Answer from the drawing. Dimensions are ordinates in mm from the lowest x, y and z of the part. Round coordinates to 2 decimals unless told otherwise and drop trailing zeros. Loops run counter-clockwise (first coordinate to the right, second up) from the corner with the lowest first, then second, coordinate; pieces in that order, holes last.
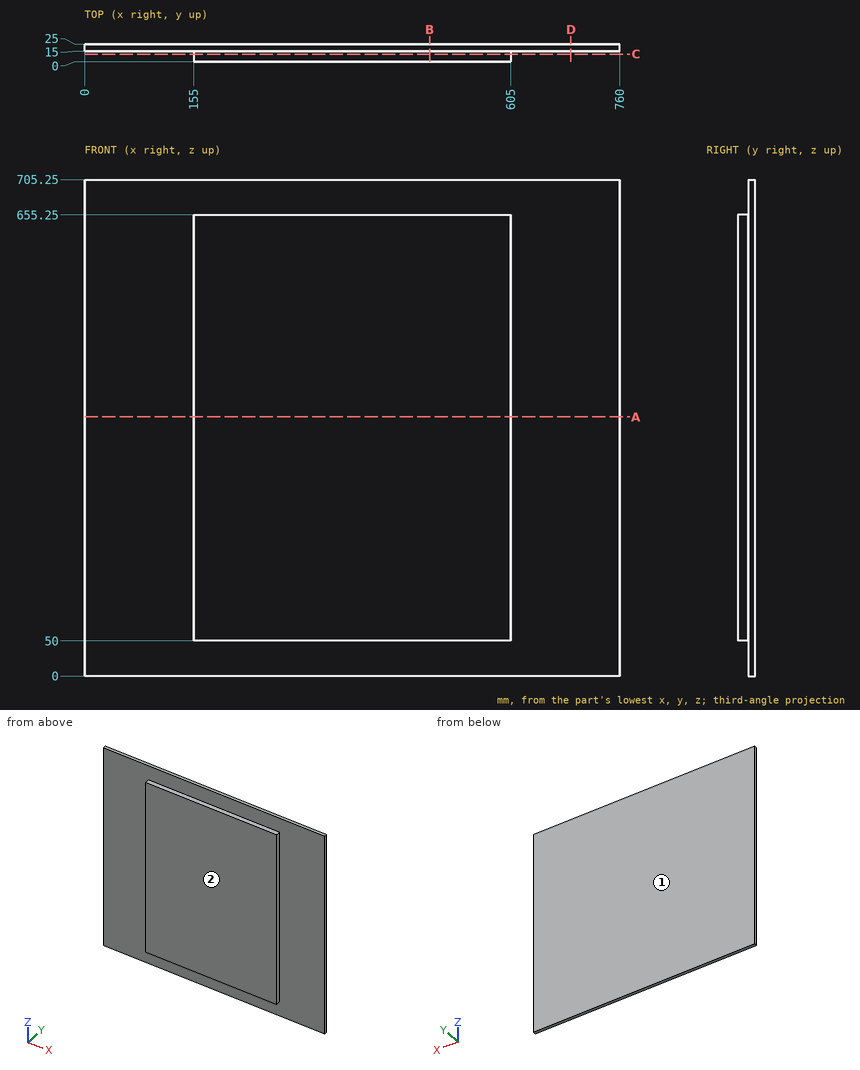
Item 1: Section C-C, the plane y = 10.5 is taken. Give the vertices of the cut face in (x, z), plus the area to 3 significant figures.
Item 2: Section D-D, the plane x = 690.5 is taken. Give the vertices of the cut face in (y, z).
Item 3: Section A-A, the plane z = 368 is taken. Give the vertices of the cut face in (x, y).
Item 4: Section B-B, the plane x = 490 is taken. Give the vertices of the cut face in (y, z).
Item 5: Straight lines are drawn through the part: line 1 (Y direction, x = 652, z = 248); line 2 (Z direction, x = 501, y = 13.75); line 3 (X direction, y = 12.25, z = 207). For each, find the intervals that lie inside material, in ascending order.
Item 6: Each of these flat-tipped pins is pushed along its axis until it touches: P1, Ø7.5, axis at x = 421, y = 5, coming from the -Z side; P2, Ø4.5, axis at y = 9, z = 481, coming from the +X side; P3, Ø10, axis at y = 7.5, z = 486.5, coming from the -X side. Where does it stop, or does it pass through?
Item 7: Determine the mould class of the marked faces 1 and 2 for opening direction Y: pulls with the +Y half, pulls with the -Y half, needs draft (parallel to the pull), parting line crosses it, or undercut.
Answer below:
1. outline: (155, 50) - (605, 50) - (605, 655.25) - (155, 655.25) - close
1. area: 272,000 mm2
2. outline: (15, 0) - (25, 0) - (25, 705.25) - (15, 705.25) - close
3. outline: (0, 15) - (155, 15) - (155, 0) - (605, 0) - (605, 15) - (760, 15) - (760, 25) - (0, 25) - close
4. outline: (0, 50) - (15, 50) - (15, 0) - (25, 0) - (25, 705.25) - (15, 705.25) - (15, 655.25) - (0, 655.25) - close
5. line 1: y = 15 to 25
5. line 2: z = 50 to 655.25
5. line 3: x = 155 to 605
6. P1: stops at z = 50
6. P2: stops at x = 605
6. P3: stops at x = 155
7. face 1: pulls with the +Y half
7. face 2: pulls with the -Y half
